Can you work these out from the model? Positions are in its coordinate system, mm. Round coordinates to 2 decimals unless told otherwise and drop trailing zeros. Loops run counter-clockwise (first coordinate to the right, second up) from the corner with the lowest first, then second, coordinate; pieces in that order, holes last.
```python
from build123d import *

# Parameters (mm, degrees)
F0_R     = 38.1
F0_R_2   = 7.5
F0_R_3   = 6
F0_R_4   = 1.55
F1_DEPTH = 5
F2_DEPTH = 25
F3_COUNT = 6
F4_DEPTH = 25
F5_COUNT = 4
F6_DEPTH = 5


with BuildPart() as f1:
    # F0 (on Top) → F1 (new body)
    with BuildSketch(Plane.XY):
        Circle(F0_R)
        Circle(F0_R_2, mode=Mode.SUBTRACT)
        with Locations((0, 20)):
            Circle(F0_R_3, mode=Mode.SUBTRACT)
        with Locations((0, 35)):
            Circle(F0_R_4, mode=Mode.SUBTRACT)
        with Locations((0, 20)):
            Circle(F0_R_3)
        with Locations((0, 35)):
            Circle(F0_R_4)
    extrude(amount=F1_DEPTH)

    # F3: F2 ×6 about axis
    f3_axis = Axis((0, 0, 5), (0, 0, 1))


with BuildPart() as f2:
    # F0 (on Top) → F2 (new body)
    with BuildSketch(Plane.XY):
        with Locations((0, 20)):
            Circle(F0_R_3)
    extrude(amount=F2_DEPTH)


with BuildPart() as f1_1:
    add(f1.part)
    for i in range(1, F3_COUNT):
        add(f2.part.rotate(f3_axis, i * 360 / F3_COUNT), mode=Mode.SUBTRACT)

    # F3#seed: cut F2
    add(f2.part, mode=Mode.SUBTRACT)

    # F5: F4 ×4 about axis
    f5_axis = Axis((0, 0, 5), (0, 0, 1))


with BuildPart() as f4:
    # F0 (on Top) → F4 (new body)
    with BuildSketch(Plane.XY):
        with Locations((0, 35)):
            Circle(F0_R_4)
    extrude(amount=F4_DEPTH)


with BuildPart() as f1_2:
    add(f1_1.part)
    for i in range(1, F5_COUNT):
        add(f4.part.rotate(f5_axis, i * 360 / F5_COUNT), mode=Mode.SUBTRACT)

    # F5#seed: cut F4
    add(f4.part, mode=Mode.SUBTRACT)

    # F0 (on Top) → F6 (join)
    with BuildSketch(Plane.XY):
        Circle(F0_R_2)
    extrude(amount=F6_DEPTH)


solid = f1_2.part
```
(1) If I drill on line 1 (Y direction, x = 0, z = 3.9); line 2 (Y direction, x = 12, z = 3.55); line 3 (Y direction, x = 16, z = 4.35), over which ranges is the centre line in solid material (lowest first)?
(2) Suppose I cut it at C-C (y = -35). Write out the boundary of the cut face in (x, z).
(3) Suppose I cut it at B-B (x = 0). Write out the boundary of the cut face in (y, z).
(4) For pin 1 (3 mm diameter, centred on y = 8, z = 1, fed in from -X), with a flat end and sliding along its axis, tell me the tip position at first contact or that it passes through.
(5) We'd pull the mould along Y, two halves only. Please class faces 1 (the cylindrical face through (12.56, -13.65, 2.46)), 2 (the flat face through (-1, 1, 0)), 3 (the cylindrical face through (-21.7, -5.9, 2.5)), 4 (the cylindrical face through (-30.235, -23.183, 2.465)): released by +Y, released by -Y, zero draft, split by the parting line, or undercut.
(6) Suppose I cut it at A-A (y = 0). Write out the boundary of the cut face in (x, z), then the cut area to 3 significant figures.
Check result:
1. line 1: y = -38.1 to -36.55, -33.45 to -26, -14 to 14, 26 to 33.45, 36.55 to 38.1
1. line 2: y = -36.16 to -12.77, -7.23 to 7.23, 12.77 to 36.16
1. line 3: y = -34.58 to -15.85, -4.15 to 4.15, 15.85 to 34.58
2. outline: (-15.05, 0) - (-1.55, 0) - (-1.55, 5) - (-15.05, 5) - close; (1.55, 0) - (15.05, 0) - (15.05, 5) - (1.55, 5) - close
3. outline: (-38.1, 0) - (-36.55, 0) - (-36.55, 5) - (-38.1, 5) - close; (-33.45, 0) - (-26, 0) - (-26, 5) - (-33.45, 5) - close; (-14, 0) - (14, 0) - (14, 5) - (-14, 5) - close; (26, 0) - (33.45, 0) - (33.45, 5) - (26, 5) - close; (36.55, 0) - (38.1, 0) - (38.1, 5) - (36.55, 5) - close
4. pin 1: stops at x = -37.54
5. face 1: undercut
5. face 2: zero draft
5. face 3: undercut
5. face 4: split by the parting line
6. outline: (-38.1, 0) - (-36.55, 0) - (-36.55, 5) - (-38.1, 5) - close; (-33.45, 0) - (33.45, 0) - (33.45, 5) - (-33.45, 5) - close; (36.55, 0) - (38.1, 0) - (38.1, 5) - (36.55, 5) - close
6. area: 350 mm2
